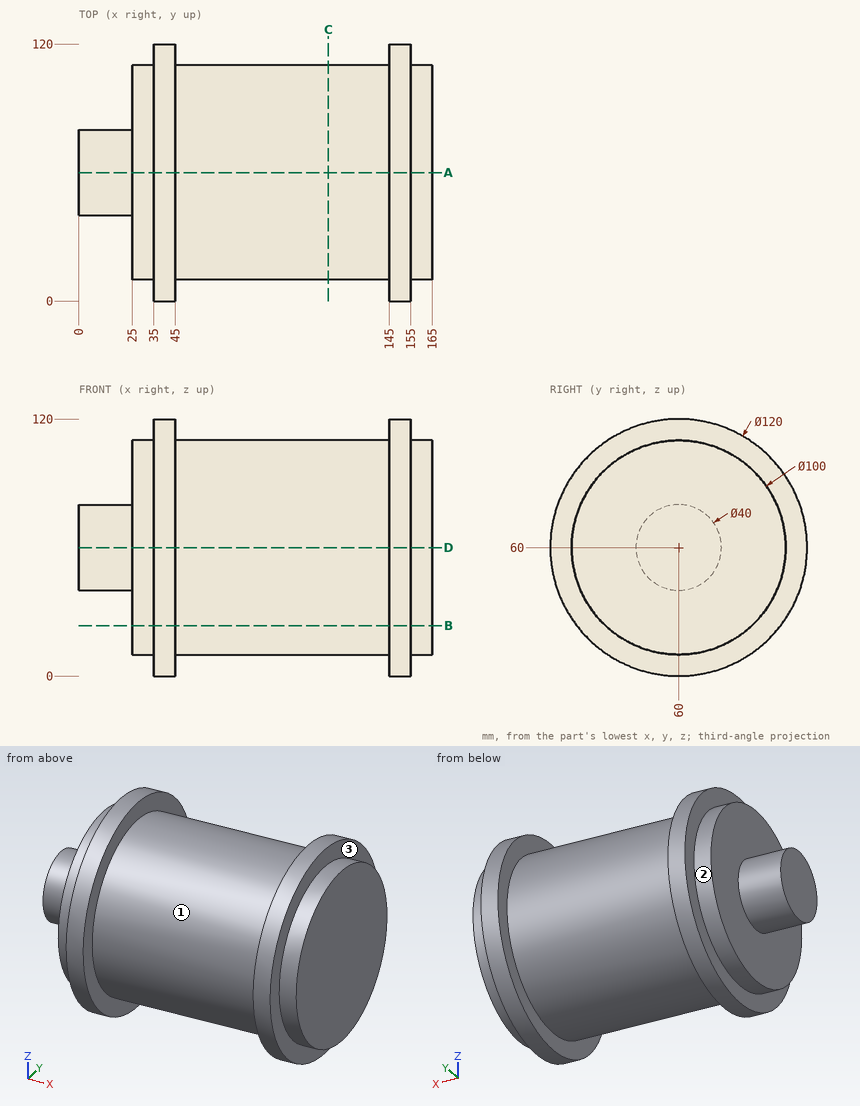
Geometry check sheet. Reference: drawing and pictorial views, mm from the part's lowest x, y, z. A direction names the side the tool comes from. Coordinates: 2 decimals unless noted, no trailing zeros. Loops run counter-clockwise (first coordinate to the right, second up) from the corner with the lowest first, then second, coordinate; pieces in that order, holes last. Notation, with made-up numbers: (71.5, 72.25) -> (96.5, 72.25) arc R34 ccw to (96.5, 110.25) -> close; hole circle Ø2 at (-28, 19). An arc over 180 degrees is marked (long way). Write item = value, one per line. Start each with the question number.
1. Material ranges on line 1 (X direction, y = 115.5, z = 65.5); line 2 (X direction, y = 55.5, z = 87); line 3 (Y direction, x = 8, z = 59), recorded low to high.
2. Section check C-C on x = 116.5. Record the cut outline in (y, z).
3. Section check A-A on y = 60. Record the cut outline in (x, z).
4. Depth check by flat-ended pin: P1, Ø10, axis at x = 58, y = 97, coming from the -Z side; P2, Ø3, axis at y = 18.5, z = 44, coming from the -X side; P3, Ø3, axis at x = 99.5, z = 65.5, coming from the +Y side; P4, Ø6, axis at x = 21, y = 106, coming from the -Z side. Enter the tip coordinate at first touch or a pass-through.
5. Section check B-B on z = 23.5. Record the cut outline in (x, y).
6. Tool access check on the marked faces 1, 2 and 3. Record the directions out of +Z, -Z, +X, -X, +Y, -Y that give a thin tool (end or side, any length) a straight path to the whole face; none if there is none.
Responses:
q1.line_1 = 35 to 45, 145 to 155
q1.line_2 = 25 to 165
q1.line_3 = 40.03 to 79.97
q2.outline = circle Ø100 at (60, 60)
q3.outline = (0, 40) -> (25, 40) -> (25, 10) -> (35, 10) -> (35, 0) -> (45, 0) -> (45, 10) -> (145, 10) -> (145, 0) -> (155, 0) -> (155, 10) -> (165, 10) -> (165, 110) -> (155, 110) -> (155, 120) -> (145, 120) -> (145, 110) -> (45, 110) -> (45, 120) -> (35, 120) -> (35, 110) -> (25, 110) -> (25, 80) -> (0, 80) -> close
q4.P1 = 21.58
q4.P2 = 25
q4.P3 = 109.84
q4.P4 = through
q5.outline = (25, 25.83) -> (35, 25.83) -> (35, 12.38) -> (45, 12.38) -> (45, 25.83) -> (145, 25.83) -> (145, 12.38) -> (155, 12.38) -> (155, 25.83) -> (165, 25.83) -> (165, 94.17) -> (155, 94.17) -> (155, 107.62) -> (145, 107.62) -> (145, 94.17) -> (45, 94.17) -> (45, 107.62) -> (35, 107.62) -> (35, 94.17) -> (25, 94.17) -> close
q6.face_1 = none
q6.face_2 = -X
q6.face_3 = +X
